```python
from build123d import *

# Parameters (mm, degrees)
SKETCH1_W           = 544
SKETCH1_H           = 107
BOSS_EXTRUDE1_DEPTH = 3
SKETCH2_W           = 30
SKETCH2_H           = 3
CUT_EXTRUDE1_DEPTH  = 3
CUT_EXTRUDE2_DEPTH  = 3
SKETCH5_W           = 3
SKETCH5_H           = 20
BOSS_EXTRUDE2_DEPTH = 3


with BuildPart() as part:
    # Sketch1 → Boss-Extrude1 (new body)
    with BuildSketch(Plane(origin=(0, 0, 0), x_dir=(1, 0, 0), z_dir=(0, 1, 0))):
        Rectangle(SKETCH1_W, SKETCH1_H)
    extrude(amount=BOSS_EXTRUDE1_DEPTH)

    # Sketch2 → Cut-Extrude1 (cut)
    with BuildSketch(Plane(origin=(0, 3, 0), x_dir=(1, 0, 0), z_dir=(0, 1, 0))):
        with Locations((62, -35)):
            Rectangle(SKETCH2_W, SKETCH2_H)
        with Locations((122, -35)):
            Rectangle(SKETCH2_W, SKETCH2_H)
        with Locations((182, -35)):
            Rectangle(SKETCH2_W, SKETCH2_H)
        with Locations((242, -35)):
            Rectangle(SKETCH2_W, SKETCH2_H)
        with Locations((-62, -35)):
            Rectangle(SKETCH2_W, SKETCH2_H)
        with Locations((-122, -35)):
            Rectangle(SKETCH2_W, SKETCH2_H)
        with Locations((-182, -35)):
            Rectangle(SKETCH2_W, SKETCH2_H)
        with Locations((-242, -35)):
            Rectangle(SKETCH2_W, SKETCH2_H)
    extrude(amount=-CUT_EXTRUDE1_DEPTH, mode=Mode.SUBTRACT)

    # Sketch4 → Cut-Extrude2 (cut)
    with BuildSketch(Plane(origin=(0, 3, 0), x_dir=(1, 0, 0), z_dir=(0, 1, 0))):
        Polygon((-164.324573519, 19.5), (-165.91228676, 22.25), (-169.08771324, 22.25), (-170.675426481, 19.5), (-169.08771324, 16.75), (-165.91228676, 16.75), align=None)
        Polygon((-164.324573519, -24.5), (-165.91228676, -21.75), (-169.08771324, -21.75), (-170.675426481, -24.5), (-169.08771324, -27.25), (-165.91228676, -27.25), align=None)
        Polygon((-70.675426481, 19.5), (-69.08771324, 16.75), (-65.91228676, 16.75), (-64.324573519, 19.5), (-65.91228676, 22.25), (-69.08771324, 22.25), align=None)
        Polygon((-70.675426481, -24.5), (-69.08771324, -27.25), (-65.91228676, -27.25), (-64.324573519, -24.5), (-65.91228676, -21.75), (-69.08771324, -21.75), align=None)
    extrude(amount=-CUT_EXTRUDE2_DEPTH, mode=Mode.SUBTRACT)

    # Sketch5 → Boss-Extrude2 (add)
    with BuildSketch(Plane(origin=(0, 0, 0), x_dir=(1, 0, 0), z_dir=(0, 1, 0))):
        with Locations((-273.5, 10)):
            Rectangle(SKETCH5_W, SKETCH5_H)
        with Locations((-273.5, -20)):
            Rectangle(SKETCH5_W, SKETCH5_H)
        with Locations((-273.5, 40)):
            Rectangle(SKETCH5_W, SKETCH5_H)
    boss_extrude2 = extrude(amount=BOSS_EXTRUDE2_DEPTH)

    # Mirror1: Boss-Extrude2 across plane
    add(boss_extrude2.mirror(Plane(origin=(0, 0, 0), x_dir=(0, 0, 1), z_dir=(1, 0, 0))))


solid = part.part
```
Input: part model. Units: mm. Frame: model coordinates. Round coordinates to 2 decimals unless told otherwise and drop trailing zeros. Order: outer loops, then holes, each group sorted by start corner. A loop starts at its lowest first (then second) coordinate and runs counter-clockwise, first axis right, second up. Notation, with made-up numbers: (-13, 59.5) - (9, 59.5) arc R11 cw to (9, 71.5) - close; hole circle Ø4 at (8, 68.25). An arc over 180 degrees is marked (long way). One line per question, with ' | ' between items. Start each with the question number.
1) Contact query for flat-ended pins moving along their axis: P1, Ø0.9, axis at y = 1.5, z = 6.5, coming from the +X side; P2, Ø0.9, axis at x = 274, y = 1.5, coming from the +Z side; P3, Ø1.5, axis at y = 1.5, z = 35, coming from the -X side. Output: stop coordinate, or through.
2) Cut plane B-B, the plane y = 2.55. Give the number of separate pieces and of enclosed holes in the cut face, then the cut area to 3 significant figures.
3) Ray query, probe 1 along Z at (x, y) = (121.5, 2.85); probe 2 along X at (y, z) = (0.4, 48). Return the intervals inside material, ascending.
4) Cut plane A-A, the plane x = 237.5. Return the cut outline in (y, z).
Worked out:
1) P1: stops at x = 272 | P2: stops at z = 30 | P3: stops at x = -272
2) separate pieces: 1 | enclosed holes: 12 | area: 57,700 mm^2
3) probe 1: z = -53.5 to 33.5, 36.5 to 53.5 | probe 2: x = -272 to 272
4) outline: (0, -53.5) - (3, -53.5) - (3, 33.5) - (0, 33.5) - close; (0, 36.5) - (3, 36.5) - (3, 53.5) - (0, 53.5) - close
